from build123d import *

# Parameters (mm, degrees)
F0_R     = 3.81
F0_R_2   = 15.24
F1_DEPTH = 3.81


with BuildPart() as f1:
    # F0 (on Front) → F1 (new body, symmetric)
    with BuildSketch(Plane.XZ):
        with BuildLine():
            ThreePointArc((5.984613, 38.451618), (8.131276, 41.431877), (8.89, 45.025544))
            ThreePointArc((8.89, 45.025544), (-3.593667, 53.156821), (-5.984613, 38.451618))
            Line((-5.984613, 38.451618), (5.984613, 38.451618))
        make_face()
        with Locations((0, 45.025544)):
            Circle(F0_R, mode=Mode.SUBTRACT)
        with BuildLine():
            ThreePointArc((5.984613, 38.451618), (0, 36.135544), (-5.984613, 38.451618))
            Line((-5.984613, 38.451618), (-11.581744, -33.278676))
            ThreePointArc((-11.581744, -33.278676), (0, -29.002925), (11.581744, -33.278676))
            Line((11.581744, -33.278676), (5.984613, 38.451618))
        make_face()
        with BuildLine():
            Line((5.984613, 38.451618), (-5.984613, 38.451618))
            ThreePointArc((-5.984613, 38.451618), (0, 36.135544), (5.984613, 38.451618))
        make_face()
        with BuildLine():
            ThreePointArc((17.823636, -46.826562), (17.194227, -42.131822), (15.350451, -37.768654))
            ThreePointArc((15.350451, -37.768654), (13.651951, -35.367667), (11.581744, -33.278676))
            ThreePointArc((11.581744, -33.278676), (0, -29.002925), (-11.581744, -33.278676))
            Line((-11.581744, -33.278676), (-15.350451, -37.768654))
            ThreePointArc((-15.350451, -37.768654), (-4.69474, -64.020789), (17.823636, -46.826562))
        make_face()
        with Locations((0, -46.826562)):
            Circle(F0_R_2, mode=Mode.SUBTRACT)
    extrude(amount=F1_DEPTH, both=True)


solid = f1.part
Part model, mm, in its own coordinate system. A direction names the side the tool comes from. Give positions to 0.01 mm unless a question says otherwise; leave off trailing zeros. Order: outer loops, then holes, each group sorted by start corner. A loop starts at its lowest first (then second) coordinate and runs counter-clockwise, first axis right, second up. Notation, with made-up numbers: (-7, 2) -> (0, 2) arc R8 ccw to (0, 7) -> close; hole circle Ø6 at (-40, 59). An arc over 180 degrees is marked (long way). Use one line per item in the form item = value.
(1) Saw through at C-C (z = -50.5). Write the cut outline in (x, y), then the cut area to 3 significant figures.
Solution:
outline = (-17.44, -3.81) -> (-14.79, -3.81) -> (-14.79, 3.81) -> (-17.44, 3.81) -> close; (14.79, -3.81) -> (17.44, -3.81) -> (17.44, 3.81) -> (14.79, 3.81) -> close
area = 40.4 mm²
(2) Saw through at D-D (x = -7). Write the cut outline in (y, z).
Solution:
outline = (-3.81, -63.22) -> (3.81, -63.22) -> (3.81, -60.36) -> (-3.81, -60.36) -> close; (-3.81, -33.29) -> (3.81, -33.29) -> (3.81, 25.44) -> (-3.81, 25.44) -> close; (-3.81, 39.55) -> (3.81, 39.55) -> (3.81, 50.51) -> (-3.81, 50.51) -> close
(3) Flat gauge pins, fed straight in: P1, Ø1.5, axis at y = 0, z = 18.5, coming from the -X side; P2, Ø18.5, axis at x = 0, z = -46.83, coming from the -Y side; P3, Ø1, axis at x = -13.5, y = -1, coming from the +Z side; P4, Ø2, axis at y = -2, z = -27, coming from the +X side. Where does each tip first touch, or does it go through?
Solution:
P1 = -7.6
P2 = through
P3 = -34.97
P4 = 11.17
(4) Tool access for faces 1 (the face through (-13.44, -0.05, -35.49)), 2 (the face through (-8.744, -0.053, 3.089)): list every direction of +Z, -Z, +X, -X, +Y, -Y with a clear straight run to the whole face (end or side of a thin tool).
Solution:
face_1 = +Z, -X, +Y, -Y
face_2 = -X, +Y, -Y
(5) Saw through at B-B (y = -2.5). Write the cut outline in (x, z), then the cut area to 3 significant figures.
Solution:
outline = (-15.35, -37.77) arc R17.82 ccw (long way) to (17.82, -46.83) arc R17.82 ccw to (15.35, -37.77) arc R17.82 ccw to (11.58, -33.28) -> (5.98, 38.45) arc R8.89 ccw to (8.89, 45.03) arc R8.89 ccw (long way) to (-5.98, 38.45) -> (-11.58, -33.28) -> close; hole circle Ø30.48 at (0, -46.83); hole circle Ø7.62 at (0, 45.03)
area = 1,640 mm²
(6) Drill centre lines: line 1 (Z direction, x = 0, y = -0.5); line 2 (Z direction, x = -5, y = -2.75); line 3 (Z direction, x = 12.5, y = -3). Where is each one in solid material? Low to high. Write a range as from..to.
Solution:
line_1 = -64.65..-62.07, -31.59..41.22, 48.84..53.92
line_2 = -63.93..-61.22, -32.43..52.38
line_3 = -59.53..-55.54, -38.11..-34.12
(7) Pull direction X, two halves, no side cores. Call faces 3 (the face through (-0.496, 0.053, 48.803)), 4 (the face through (0, -3.81, -5)), 5 (the face through (8.822, -0.053, 2.084)): +X half, -X half, draft (parallel to the pull), parting line (faces both ways), or undercut.
Solution:
face_3 = undercut
face_4 = draft
face_5 = +X half
(8) Saw through at A-A (x = 0). Write the cut outline in (y, z), then the cut area to 3 significant figures.
Solution:
outline = (-3.81, -64.65) -> (3.81, -64.65) -> (3.81, -62.07) -> (-3.81, -62.07) -> close; (-3.81, -31.59) -> (3.81, -31.59) -> (3.81, 41.22) -> (-3.81, 41.22) -> close; (-3.81, 48.84) -> (3.81, 48.84) -> (3.81, 53.92) -> (-3.81, 53.92) -> close
area = 613 mm²
